Autodesk Inventor part; units mm, degrees
ref_plane "YZ Plane" through (0, 0, 0) normal (1, 0, 0) x (0, 1, 0)
ref_plane "XZ Plane" through (0, 0, 0) normal (0, 1, 0) x (-1, 0, 0)
ref_plane "XY Plane" through (0, 0, 0) normal (0, 0, 1) x (1, 0, 0)
sketch "Sketch1" plane through (0, 0, 0) normal (1, 0, 0) x (0, 1, 0)
  line L0 (0, 0) -> (8, 0)
  line L1 (8, 0) -> (8, 30)
  line L2 (8, 30) -> (0, 30)
  line L3 (0, 30) -> (0, 0)
  line L4 (8, 10) -> (4, 10)
  line L5 (4, 10) -> (4, 20)
  line L6 (4, 20) -> (8, 20)
  line L7 (8, 20) -> (8, 10)
  dimension "d0" = 8
  dimension "d1" = 30
  dimension "d2" = 4
  dimension "d3" = 10
  dimension "d4" = 10
extrude "Extrusion1" add sketch "Sketch1" against normal blind 8 contours L3 L2 L1 L6 L5 L4 L0
sketch "Sketch2" plane through (0, 4, 20) normal (0, 1, 0) x (1, 0, 0)
  line L0 (0, 10) -> (0, 0)
  line L1 (0, 10) -> (-8, 10)
  line L2 (-8, 0) -> (-8, 10)
  line L3 (0, 0) -> (-8, 0)
  line L4 (-8, 0) -> (0, 10) construction
  line L5 (-8, 10) -> (0, 0) construction
  circle A0 centre (-4, 5) radius 2.75
  point P0 (0, 20)
  dimension "d7" = 5.5
extrude "Extrusion2" cut sketch "Sketch2" against normal up to next contours A0
sketch "Sketch3" plane through (0, 0, 0) normal (1, 0, 0) x (0, 0, -1)
  line L0 (0, 8) -> (-10, 8)
  line L1 (-10, 8) -> (-10, 4)
  line L2 (-10, 4) -> (-20, 4)
  line L3 (-20, 4) -> (-20, 8)
  line L4 (-20, 8) -> (-30, 8)
  line L5 (-30, 8) -> (-30, 0)
  line L6 (-30, 0) -> (0, 0)
  line L7 (0, 0) -> (0, 8)
  line L8 (-8, 7) -> (-2, 7)
  line L9 (-2, 7) -> (-2, 5)
  line L10 (-2, 5) -> (-8, 5)
  line L11 (-8, 5) -> (-8, 7)
  line L12 (-20, 4) -> (-10, 4) construction
  line L13 (-15, 4) -> (-15, 8) construction
  line L14 (-22, 7) -> (-28, 7)
  line L15 (-28, 7) -> (-28, 5)
  line L16 (-28, 5) -> (-22, 5)
  line L17 (-22, 5) -> (-22, 7)
  dimension "d10" = 6
  dimension "d11" = 2
  dimension "d12" = 10
  dimension "d13" = 2
  dimension "d14" = 4
  dimension "d15" = 1
extrude "Extrusion3" cut sketch "Sketch3" against normal up to next contours L8 L9 L10 L11 | L17 L16 L15 L14
fillet "Fillet1" radius 2 8 edges at (-4, 8, 10) (-4, 8, 20) (-4, 8, 30) (-4, 8, 0) (-4, 7, 28) (-4, 7, 22) (-4, 7, 8) (-4, 7, 2)
equation "\"d4\" = -0.5 * d3 + 0.5 * d1"
equation "\"d13\" = -0.5 * d10 + 0.5 * d12"
equation "\"d15\" = -0.5 * d11 + 0.5 * d14"
properties part number "Wire Anchor"
Read the model definition and answer for the solid it produces. Units are mm, in the model's axes. A direction names the side the tool comes from. Give positions to 0.01 mm unless a question says otherwise; leave off trailing zeros. Loops run counter-clockwise (first coordinate to the right, second up) from the corner with the lowest first, then second, coordinate; pieces in that order, holes last.
Item 1: Find the intervals of material crossed by line 1 along X through (y, z) = (2.5, 15); line 2 along Z through (x, y) = (-5.25, 5.5); line 3 along Z through (x, y) = (-4, 2.7), in increasing order.
Item 2: For faces 4 (the flat face through (-4, 7, 5)), 5 (the flat face through (-8, 3, 15)), 6 (the cylindrical face through (-4.06, 7.43, 20.6)), determine the directions among +Z, -Z, +X, -X, +Y, -Y from which every point of the face is accessible in a straight line to the end or side of a thin tool.
Item 3: The part is cut by section C-C (y = 5.5). Write down the section's boundary in (x, z).
Item 4: Each of these flat-tipped pins is pushed along its axis until it touches: pin 1 Ø4 at (x, z) = (-3, 14) entering from +Y; pin 2 Ø1.5 at (x, z) = (-2.5, 21) entering from +Y. Where does it stop, or does it pass through?
Item 5: The part is cut by section B-B (z = 15). Write down the section's boundary in (x, y).
Item 6: The part is cut by section D-D (y = 0.5). Write down the section's boundary in (x, z).
Item 7: The mould has two halves that part along Y. Classify faces 1 (the flat face through (-4, 0, 19)), 2 (the cylindrical face through (-4.06, 6.4, 7.43)), 3 (the flat face through (-4, 5, 20)): released by +Y, released by -Y, zero draft, split by the parting line, or undercut.
Item 8: The part is cut by section A-A (x = -4). Give the number of separate pieces and of enclosed holes in the cut face, and give its area (3 significant figures).
Taken from the geometry:
1. line 1: x = -8 to -6.75, -1.25 to 0
1. line 2: z = 0 to 2.06, 7.94 to 10, 20 to 22.06, 27.94 to 30
1. line 3: z = 0 to 12.25, 17.75 to 30
2. face 4: +X, -X
2. face 5: +Z, -Z, -X, +Y, -Y
2. face 6: +X, -X, +Y
3. outline: (-8, 0) - (0, 0) - (0, 2.06) - (-8, 2.06) - close; (-8, 7.94) - (0, 7.94) - (0, 10) - (-8, 10) - close; (-8, 20) - (0, 20) - (0, 22.06) - (-8, 22.06) - close; (-8, 27.94) - (0, 27.94) - (0, 30) - (-8, 30) - close
4. pin 1: stops at y = 4
4. pin 2: stops at y = 7.98
5. outline: (-8, 0) - (-6.75, 0) - (-6.75, 4) - (-8, 4) - close; (-1.25, 0) - (0, 0) - (0, 4) - (-1.25, 4) - close
6. outline: (-8, 0) - (0, 0) - (0, 30) - (-8, 30) - close; hole circle Ø5.5 at (-4, 15)
7. face 1: released by -Y
7. face 2: undercut
7. face 3: zero draft
8. separate pieces: 2
8. enclosed holes: 2
8. area: 154 mm2
